Part print with two shaded views. Sizes in mm from the minimum x, y, z corner. A direction names the side the tool comes from. Coordinates: 2 decimals unless noted, no trailing zeros. Order: outer loops, then holes, each group sorted by start corner. A loop starts at its lowest first (then second) coordinate and runs counter-clockwise, first axis right, second up. Notation, with made-up numbers: (72, 79) - (111, 79) arc R25 ccw to (111, 118) - close; hole circle Ø11 at (79.5, -20). An arc over 180 degrees is marked (long way). Return JSON: item names as keys, results as strings.
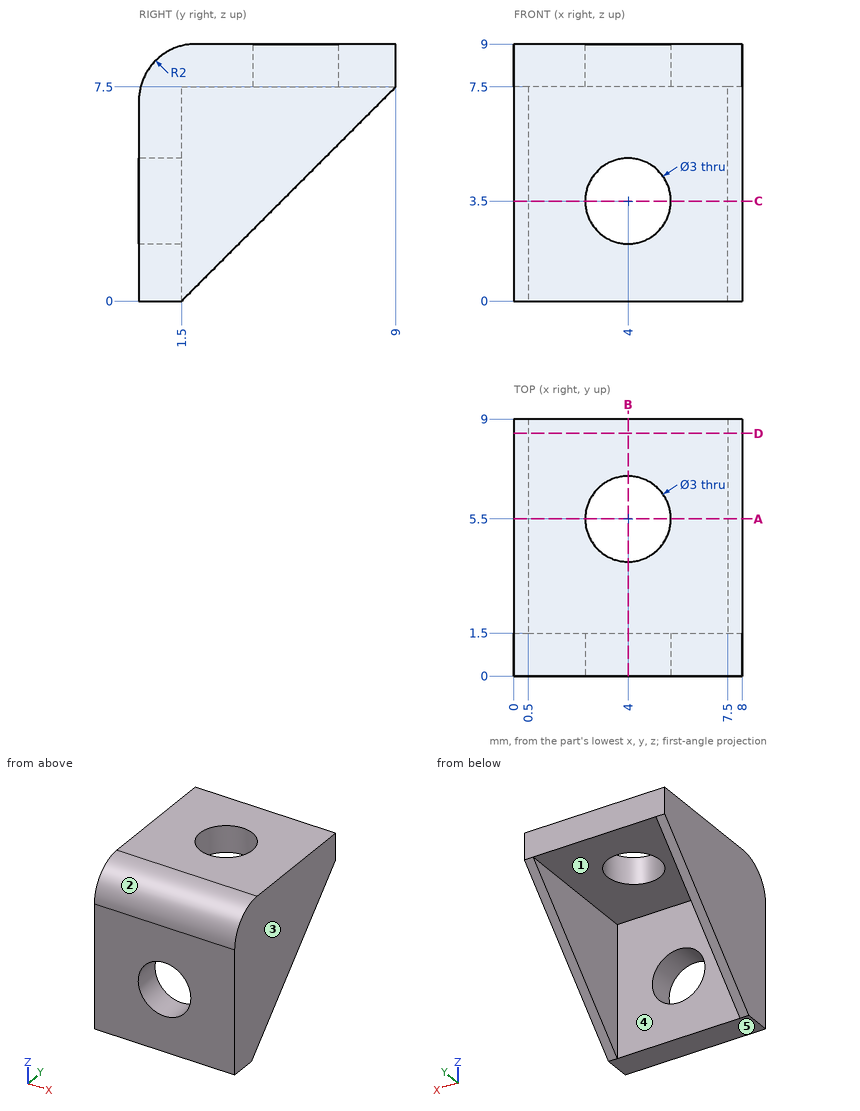
Item 1: Which spindle directions (+Z, -Z, +X, -X, +Y, -Y) get a long thin tool onto all of the face, cutting with end or side? Do the marked faces 4 and 5. Say none if no direction does.
Findings below:
{"face 4": "-Z, +Y", "face 5": "-Z, +X, -X, +Y, -Y"}
Item 2: Drop flat-ended pins along their axis: P1, Ø3.5, axis at x = 5.5, z = 2, coming from the +Y side; P2, Ø1.5, axis at x = 5, y = 5, coming from the -Z side. Give the stop position or say it passes through.
Findings below:
{"P1": "stops at y = 1.5", "P2": "stops at z = 7.5"}
Item 3: Mould opens along X. For the marked faces 1, 2 and 3 say: released by +X, released by -X, zero draft, split by the parting line, or undercut.
Findings below:
{"face 1": "undercut", "face 2": "zero draft", "face 3": "released by +X"}
Item 4: Band-saw the part on C-C, the plane z = 3.5. List the corners of the cut face in (x, y), then the cut area to 3 significant figures.
Findings below:
{"outline": "(0, 0) - (2.5, 0) - (2.5, 1.5) - (0.5, 1.5) - (0.5, 5) - (0, 5) - close; (5.5, 0) - (8, 0) - (8, 5) - (7.5, 5) - (7.5, 1.5) - (5.5, 1.5) - close", "area": "11.0 mm²"}
Item 5: Band-saw the part on A-A, the plane y = 5.5. List the corners of the cut face in (x, z).
Findings below:
{"outline": "(0, 4) - (0.5, 4) - (0.5, 7.5) - (2.5, 7.5) - (2.5, 9) - (0, 9) - close; (5.5, 7.5) - (7.5, 7.5) - (7.5, 4) - (8, 4) - (8, 9) - (5.5, 9) - close"}
Item 6: Wall check: L1, parallel to X at y = 3, z = 6; L2, parallel to X at y = 0.35, z = 3.5; L3, parallel to Y at x = 4, z = 8.2. Give the ranges that are in metal, low to high. Write a range as [from, to].
Findings below:
{"L1": "x = [0, 0.5], [7.5, 8]", "L2": "x = [0, 2.5], [5.5, 8]", "L3": "y = [0.4, 4], [7, 9]"}
Item 7: Band-saw the part on B-B, the plane x = 4. List the corners of the cut face in (y, z), then the cut area to 3 significant figures.
Findings below:
{"outline": "(0, 0) - (1.5, 0) - (1.5, 2) - (0, 2) - close; (0, 5) - (1.5, 5) - (1.5, 7.5) - (4, 7.5) - (4, 9) - (2, 9) arc R2 ccw to (0, 7) - close; (7, 7.5) - (9, 7.5) - (9, 9) - (7, 9) - close", "area": "14.9 mm²"}
Item 8: Band-saw the part on D-D, the plane y = 8.5. List the corners of the cut face in (x, z), then the cut area to 3 significant figures.
Findings below:
{"outline": "(0, 7) - (0.5, 7) - (0.5, 7.5) - (7.5, 7.5) - (7.5, 7) - (8, 7) - (8, 9) - (0, 9) - close", "area": "12.5 mm²"}
